Build history of the part. All positions in model axes, mm. A direction names the side the tool comes from. Coordinates: 2 decimals unless noted, no trailing zeros. Loops run counter-clockwise (first coordinate to the right, second up) from the corner with the lowest first, then second, coordinate; pieces in that order, holes last.
(1) Two-plate mould, pull along Z, no slides. Class faces 3 (the face through (-22, -311, 0)), 4 (the face through (0, -311, -25)), 5 (the face through (0.1, -24.9, -22.3)): pulls with the +Z half, pulls with the -Z half, needs draft (parallel to the pull), parting line crosses it, or undercut.
(2) Slice it at B-B (x = 6). Give the cut face in (y, z), and give its area (3 significant figures).
(3) Slice it at A-A (z = 7). Give the cut face in (x, y), and give its area (3 significant figures).
(4) Flat gauge pins, fed straight in: P1, Ø6, axis at x = 17, z = -2, coming from the -Y side; P2, Ø12, axis at x = 15, z = 18, coming from the +Y side. Where does each tip first touch, or does it go through?
(5) Slice it at C-C (y = -131.5). Give the cut face in (x, z).
(6) Tool access for faces 1 (the face through (-25, -311, 0)), 2 (the face through (0, -311, -22)): list every direction of +Z, -Z, +X, -X, +Y, -Y with a clear straight run to the whole face (end or side of a thin tool).
(7) Wall check: L1, parallel to Z at x = -5.5, y = -71; L2, parallel to X at y = -26, z = -15. Give the ranges that are in metal, low to high.
from build123d import *

# Parameters (mm, degrees)
F0_W        = 50
F0_H        = 50
F0_W_2      = 44
F0_H_2      = 44
F1_DEPTH    = 630
F2_T1_DEPTH = 307.1682987966
F3_T1_DEPTH = 307.1682987966


# Not quite as in the source:
# - a fillet or chamfer that OpenCascade refuses, or shapes differently, is made with other operations: its cross-section is extruded or revolved along the edge and cut away or added


with BuildPart() as f1:
    # F0 (on Front) → F1 (new body)
    with BuildSketch(Plane.XZ):
        Rectangle(F0_W, F0_H)
        Rectangle(F0_W_2, F0_H_2, mode=Mode.SUBTRACT)
    extrude(amount=F1_DEPTH)

    # F2: chamfer of 50 on 1 edges, made by hand

    # F2_s2 → F2_t1 (cut)
    with BuildSketch(Plane.XY.offset(-153.5841493983)):
        Polygon((-25, -580), (25, -630), (-25, -630), align=None)
    extrude(amount=F2_T1_DEPTH, mode=Mode.SUBTRACT)

    # F3: chamfer of 50 on 1 edges, made by hand

    # F3_s2 → F3_t1 (cut)
    with BuildSketch(Plane.XY.offset(-153.5841493983)):
        Polygon((25, 0), (-25, -50), (-25, 0), align=None)
    extrude(amount=F3_T1_DEPTH, mode=Mode.SUBTRACT)


solid = f1.part
Response values:
1. face 3: undercut
1. face 4: pulls with the -Z half
1. face 5: needs draft
2. outline: (-611, -25) - (-19, -25) - (-19, -22) - (-611, -22) - close; (-611, 22) - (-19, 22) - (-19, 25) - (-611, 25) - close
2. area: 3,550 mm2
3. outline: (-25, -580) - (-22, -583) - (-22, -47) - (-25, -50) - close; (22, -627) - (25, -630) - (25, 0) - (22, -3) - close
3. area: 3,480 mm2
4. P1: passes through
4. P2: stops at y = -5.53
5. outline: (-25, -25) - (25, -25) - (25, 25) - (-25, 25) - close; hole (-22, -22) - (22, -22) - (22, 22) - (-22, 22) - close
6. face 1: +Z, -Z, -X, +Y, -Y
6. face 2: +Y, -Y
7. L1: z = -25 to -22, 22 to 25
7. L2: x = 22 to 25
